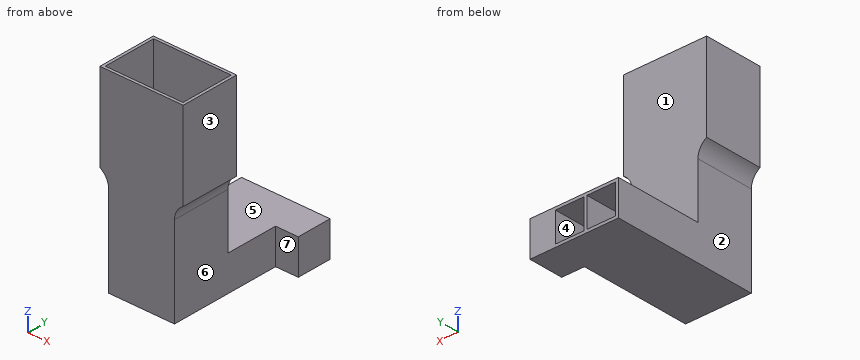
```python
from build123d import *

# Parameters (mm, degrees)
F2_W        = 18.8
F2_H        = 30
F3_DEPTH    = 16.8
F4_T1_DEPTH = 16.8
F5_T        = 0.8
F5_T3_DEPTH = 18.4
F6_W        = 18.8
F6_H        = 10
F7_DEPTH    = 25
F8_T        = -0.8
F9_DEPTH    = 0.8
F10_W       = 0.8
F10_H       = 8.4
F11_DEPTH   = 25.8
F12_W       = 10
F12_H       = 10
F13_DEPTH   = 6.5


# Not quite as in the source:
# - a fillet or chamfer that OpenCascade refuses, or shapes differently, is made with other operations: its cross-section is extruded or revolved along the edge and cut away or added
# - a shell that OpenCascade refuses in one call is made with other operations: the cavity is built on its own and cut out


with BuildPart() as f3:
    # F2 (on Front) → F3 (new body)
    with BuildSketch(Plane.XZ):
        Polygon((23.8, 25), (0, 25), (0, 0), (2.5, 0), (21.3, 0), (23.8, 0), align=None)
        with Locations((11.9, -15)):
            Rectangle(F2_W, F2_H)
    extrude(amount=F3_DEPTH)

    # F4: fillet of radius 5 on 2 edges, made by hand

    # F4_s2 → F4_t1 (join)
    with BuildSketch(Plane.XZ):
        with BuildLine():
            ThreePointArc((0.0002000386, 0.0003463879), (1.8304834454, -1.8302431314), (2.5004, -4.3306845218))
            Line((2.5004, -4.3306845218), (3.0005365685, -4.3306845218))
            ThreePointArc((3.0005365685, -4.3306845218), (3.0001365685, -2.1653422609), (3.0001365685, 0))
            Line((3.0001365685, 0), (2.5, 0.5001365685))
            ThreePointArc((2.5, 0.5001365685), (1.2501000193, 0.5001365685), (0.250316611, 0.4334494788))
            Line((0.250316611, 0.4334494788), (0.0002000386, 0.0003463879))
        make_face()
        with BuildLine():
            ThreePointArc((21.2996, -4.3306845218), (21.9695165546, -1.8302431314), (23.7997999614, 0.0003463879))
            Line((23.7997999614, 0.0003463879), (23.549683389, 0.4334494788))
            ThreePointArc((23.549683389, 0.4334494788), (22.5498999807, 0.5001365685), (21.3, 0.5001365685))
            Line((21.3, 0.5001365685), (20.7998634315, 0))
            ThreePointArc((20.7998634315, 0), (20.7998634315, -2.1653422609), (20.7994634315, -4.3306845218))
            Line((20.7994634315, -4.3306845218), (21.2996, -4.3306845218))
        make_face()
    extrude(amount=F4_T1_DEPTH)

    # F5: shell of thickness 0.8, made by hand


with BuildPart() as f5_core1:
    # F5_t2: copy of F3
    add(f3.part)

    # the walls: a layer under each face that stays
    f5_faces = [f5_core1.faces().sort_by_distance(p)[0] for p in [
        (23.8, -8.4, 12.5),
        (0, -8.4, 12.5),
        (11.9, 0, -2.5),
        (11.9, -16.8, -2.5),
        (23.7996001251, -8.4, 0),
        (0.0003998749, -8.4, 0),
        (21.3, -8.4, -17.1337157982),
        (11.9, -8.4, -30),
        (2.5, -8.4, -17.1337157982),
        (21.9852401758, -8.4, -1.8032011796),
        (1.8147598242, -8.4, -1.8032011796),
    ]]
    thicken(f5_faces, amount=-F5_T, mode=Mode.SUBTRACT)

    # F5_s4 → F5_t3 (cut)
    with BuildSketch(Plane.XZ.offset(-0.8)):
        Polygon((23.803201982, -0.0149272032), (23.7992002503, 0.8), (23.5847337286, 0.8), (23.3990270828, 0.6927203159), align=None)
        Polygon((-0.003201982, -0.0149272032), (0.0007997497, 0.8), (0.2152662714, 0.8), (0.4009729172, 0.6927203159), align=None)
        Polygon((21.3159993602, -4.2675327735), (20.5, -4.2674315965), (20.5, -4.2623725419), (20.5000639825, -4.257313892), align=None)
        Polygon((2.4840006398, -4.2675327735), (3.3, -4.2674315965), (3.3, -4.2623725419), (3.2999360175, -4.257313892), align=None)
    extrude(amount=F5_T3_DEPTH, mode=Mode.SUBTRACT)


with BuildPart() as f3_1:
    add(f3.part)

    # what is left inside the walls is the cavity
    f5_cavity = [f5_core1.part.solids().sort_by_distance(p)[0] for p in [
        (11.9, -15.992, -11.133333),
    ]]
    add(f5_cavity, mode=Mode.SUBTRACT)

    # F6 (on face) → F7 (join)
    with BuildSketch(Plane(origin=(0, 0, 0), x_dir=(-1, 0, 0), z_dir=(0, 1, 0))):
        with Locations((-11.9, -25)):
            Rectangle(F6_W, F6_H)
    extrude(amount=F7_DEPTH)

    # F8
    f8_openings = [f3_1.faces().sort_by_distance(p)[0] for p in [
        (11.9, 25, -25),
    ]]
    offset(amount=F8_T, openings=f8_openings, kind=Kind.INTERSECTION)

    # F9 (cut, through all): a face of the model
    f9_faces = [f3_1.faces().sort_by_distance(p)[0] for p in [
        (11.9, 0, -25),
    ]]
    extrude(f9_faces, amount=-F9_DEPTH, mode=Mode.SUBTRACT)

    # F10 (on face) → F11 (join, through all)
    with BuildSketch(Plane(origin=(0, 25, 0), x_dir=(-1, 0, 0), z_dir=(0, 1, 0))):
        with Locations((-11.9, -25)):
            Rectangle(F10_W, F10_H)
    extrude(amount=-F11_DEPTH)

    # F12 (on face) → F13 (join)
    with BuildSketch(Plane.YZ.offset(21.3)):
        with Locations((20, -25)):
            Rectangle(F12_W, F12_H)
    extrude(amount=F13_DEPTH)


solid = f3_1.part
```
Could you check a few things on this model? Use its own coordinates, in mm. Face numbers are marked on the shaded views. A direction names the side the tool comes from. Coordinates: 2 decimals unless noted, no trailing zeros. Write each loop counter-clockwise with the first axis right and the second up, starting at its lowest first coordinate (ties: lowest second). Pieces come first, ordered by that corner, then holes. Notation, with made-up numbers: (72.25, -13) - (83.25, -13) arc R16 ccw to (83.25, -8) - close; hole circle Ø4 at (77.25, 10). An arc over 180 degrees is marked (long way). Use a Markdown table: item, result.
Q1. Thinking about a two-plate mould opening in X: for the marked faces 1, 2, 3 and 4, which applies, +X half, -X half, draft (parallel to the pull), parting line (faces both ways), or undercut?
Geometry check:
| item | result |
|---|---|
| face 1 | draft |
| face 2 | -X half |
| face 3 | +X half |
| face 4 | undercut |
Q2. Imagine slicing it at D-D (z = -26). List the corners of the cut face in (x, y) for me.
Geometry check:
| item | result |
|---|---|
| outline | (2.5, -16.8) - (21.3, -16.8) - (21.3, 15) - (27.8, 15) - (27.8, 25) - (20.5, 25) - (20.5, -16) - (3.3, -16) - (3.3, 25) - (2.5, 25) - close; (11.5, -0.8) - (12.3, -0.8) - (12.3, 25) - (11.5, 25) - close |
Q3. Imagine slicing it at B-B (x = 9). List the corners of the cut face in (y, z) for me.
Geometry check:
| item | result |
|---|---|
| outline | (-16.8, -30) - (25, -30) - (25, -29.2) - (-16, -29.2) - (-16, 25) - (-16.8, 25) - close; (-0.8, -20.8) - (25, -20.8) - (25, -20) - (0, -20) - (0, 25) - (-0.8, 25) - close |
Q4. I'm going to push flat-ended pins straight in: pin 1 Ø1 at (y, z) = (-3, -10.5) entering from +X; pin 2 Ø12.5 at (x, y) = (18, 16) entering from +Z; pin 3 Ø7.5 at (y, z) = (-6.5, 17.5) entering from +X. Where does each tip first touch, or does it pass through?
Geometry check:
| item | result |
|---|---|
| pin 1 | stops at x = 21.3 |
| pin 2 | stops at z = -20 |
| pin 3 | stops at x = 23.8 |
Q5. Which directions (+Z, -Z, +X, -X, +Y, -Y) give clear straight access to the entire face, cutting with the end or side of a thin tool? Please do the marked faces 5, 6 and 7.
Geometry check:
| item | result |
|---|---|
| face 5 | +Z, +X, -X, +Y |
| face 6 | -Z, +X, -Y |
| face 7 | +Z, -Z, +X, -Y |
Q6. Imagine slicing it at A-A (z = -14). List the corners of the cut face in (x, y) for me, and give its area (3 significant figures).
Geometry check:
| item | result |
|---|---|
| outline | (2.5, -16.8) - (21.3, -16.8) - (21.3, 0) - (2.5, 0) - close; hole (3.3, -16) - (20.5, -16) - (20.5, -0.8) - (3.3, -0.8) - close |
| area | 54.4 mm2 |
Q7. Please list where these lines run through material, in increasing order: L1, parallel to X at y = 16, z = -24.5; L2, parallel to Z at x = 15.25, y = 21; L3, parallel to X at y = -9, z = 12.
Geometry check:
| item | result |
|---|---|
| L1 | x = 2.5 to 3.3, 11.5 to 12.3, 20.5 to 27.8 |
| L2 | z = -30 to -29.2, -20.8 to -20 |
| L3 | x = 0 to 0.8, 23 to 23.8 |
Q8. Imagine slicing it at C-C (y = 13). List the corners of the cut face in (x, z) for me, and give its area (3 significant figures).
Geometry check:
| item | result |
|---|---|
| outline | (2.5, -30) - (21.3, -30) - (21.3, -20) - (2.5, -20) - close; hole (3.3, -29.2) - (11.5, -29.2) - (11.5, -20.8) - (3.3, -20.8) - close; hole (12.3, -29.2) - (20.5, -29.2) - (20.5, -20.8) - (12.3, -20.8) - close |
| area | 50.2 mm2 |
